Design review of the part built by this model. Coordinates are the model's own, in mm. Face numbers are marked on the shaded views. A direction names the side the tool comes from. Coordinates: 2 decimals unless noted, no trailing zeros. Order: outer loops, then holes, each group sorted by start corner. A loop starts at its lowest first (then second) coordinate and runs counter-clockwise, first axis right, second up. Notation, with made-up numbers: M 16.5,45 L 69.5,45 A16 cw 69.5,56 Z; hole C 45,-15.75 d8. An arc over 180 degrees is marked long. Use CSV: the item, a comma, the result in double quotes.
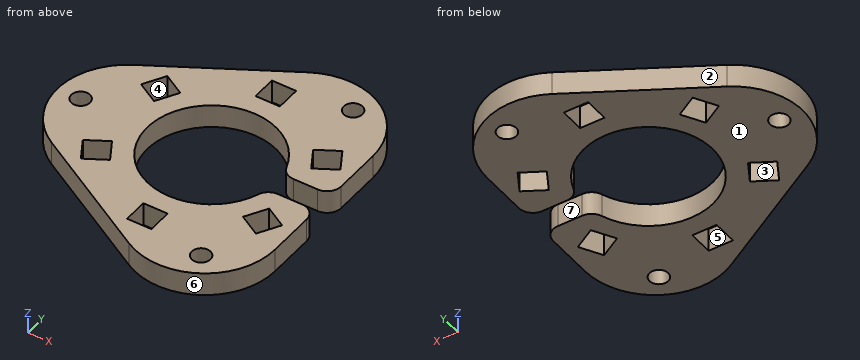
```python
from build123d import *

# Parameters (mm, degrees)
SKETCH1_R           = 2
SKETCH1_W           = 5.2
SKETCH1_H           = 5.2
BOSS_EXTRUDE1_DEPTH = 5
CONG_1_R            = 15
CONG_2_R            = 3


with BuildPart() as part:
    # Sketch1 → Boss-Extrude1 (new body)
    with BuildSketch(Plane.XY):
        with BuildLine():
            Line((24, 2.5), (13.520817283, 2.5))
            ThreePointArc((13.520817283, 2.5), (-13.75, 0), (13.520817283, -2.5))
            Line((13.520817283, -2.5), (24, -2.5))
            Line((24, -2.5), (24, -41.569219382))
            Line((24, -41.569219382), (-48, 0))
            Line((-48, 0), (24, 41.569219382))
            Line((24, 41.569219382), (24, 2.5))
        make_face()
        with Locations((14, 24.248711306)):
            Circle(SKETCH1_R, mode=Mode.SUBTRACT)
        with Locations((14, -24.248711306)):
            Circle(SKETCH1_R, mode=Mode.SUBTRACT)
        with Locations((-28, 0)):
            Circle(SKETCH1_R, mode=Mode.SUBTRACT)
        with Locations((0, 20.5)):
            Rectangle(SKETCH1_W, SKETCH1_H, mode=Mode.SUBTRACT)
        Polygon((21.305186827, 9.29833395), (16.801854728, 6.69833395), (14.201854728, 11.20166605), (18.705186827, 13.80166605), align=None, mode=Mode.SUBTRACT)
        Polygon((18.705186827, -13.80166605), (14.201854728, -11.20166605), (16.801854728, -6.69833395), (21.305186827, -9.29833395), align=None, mode=Mode.SUBTRACT)
        with Locations((0, -20.5)):
            Rectangle(SKETCH1_W, SKETCH1_H, mode=Mode.SUBTRACT)
        Polygon((-21.305186827, -9.29833395), (-16.801854728, -6.69833395), (-14.201854728, -11.20166605), (-18.705186827, -13.80166605), align=None, mode=Mode.SUBTRACT)
        Polygon((-18.705186827, 13.80166605), (-14.201854728, 11.20166605), (-16.801854728, 6.69833395), (-21.305186827, 9.29833395), align=None, mode=Mode.SUBTRACT)
    extrude(amount=BOSS_EXTRUDE1_DEPTH)

    # Congé1
    cong_1_edges = [part.edges().sort_by_distance(p)[0] for p in [
        (24, -41.569219382, 2.5),
        (-48, 0, 2.5),
        (24, 41.569219382, 2.5),
    ]]
    fillet(cong_1_edges, radius=CONG_1_R)

    # Congé2
    cong_2_edges = [part.edges().sort_by_distance(p)[0] for p in [
        (24, 2.5, 2.5),
        (13.520817283, 2.5, 2.5),
        (13.520817283, -2.5, 2.5),
        (24, -2.5, 2.5),
    ]]
    fillet(cong_2_edges, radius=CONG_2_R)


solid = part.part
```
(1) Add section B-B on x = 7.5. State the section outline as (y, z) points.
The answers:
outline,"M -30.51,0 L -11.52,0 L -11.52,5 L -30.51,5 Z; M 11.52,0 L 30.51,0 L 30.51,5 L 11.52,5 Z"
(2) Clearance check with flat-ended pins moving along their axes: P1, Ø2.5, axis at x = 1, z = 2, coming from the -Y side; P2, Ø1.5, axis at y = -20.5, z = 1.5, coming from the -X side; P3, Ø2.5, axis at x = 18.5, z = 3.5, coming from the -Y side; P4, Ø2.5, axis at x = 14, y = -24.25, coming from the +Z side. State where each tip first meets the part, or that it passes through.
The answers:
P1,"stops at y = -28.98"
P2,"stops at x = -13.79"
P3,"stops at y = -28.12"
P4,"passes through"
(3) Wall thickness on probe 1 along Y at (x, z) = (0, 1.95); probe 2 along Y at (x, z) = (-20.5, 2.6); probe 3 along Y at (x, z) = (17, 4.55): over which ranges is each line inside the solid? List them lowest first.
The answers:
probe 1,"y = -27.71 to -23.1, -17.9 to -13.75, 13.75 to 17.9, 23.1 to 27.71"
probe 2,"y = -15.88 to -10.69, -8.83 to 8.83, 10.69 to 15.88"
probe 3,"y = -28.28 to -12.82, -6.81 to -2.5, 2.5 to 6.81, 12.82 to 28.28"
(4) For the marked faces 5, 6 and 7, list the 3-axis set-ups (+Z, -Z, +X, -X, +Y, -Y) from which the entire face can be reached by the end or side of a thin tool; tool diameter is ignored.
The answers:
face 5,"+Z, -Z"
face 6,"+Z, -Z, -Y"
face 7,"+Z, -Z, +X"
(5) The part is to be moulded in two halves that separate along Y. For the marked faces 1, 2, 3 and 4, say which applies: pulls with the +Y half, pulls with the -Y half, needs draft (parallel to the pull), parting line crosses it, or undercut.
The answers:
face 1,"needs draft"
face 2,"pulls with the +Y half"
face 3,"undercut"
face 4,"undercut"
(6) Add section C-C on x = 0. State the section outline as (y, z) points.
The answers:
outline,"M -27.71,0 L -23.1,0 L -23.1,5 L -27.71,5 Z; M -17.9,0 L -13.75,0 L -13.75,5 L -17.9,5 Z; M 13.75,0 L 17.9,0 L 17.9,5 L 13.75,5 Z; M 23.1,0 L 27.71,0 L 27.71,5 L 23.1,5 Z"
(7) Add section D-D on z = 1.05. Give the number of separate pieces and of enclosed holes in the cut face, and give its area (3 significant figures).
The answers:
separate pieces,"1"
enclosed holes,"9"
area,"1,680 mm2"
(8) Add section A-A on y = 0. State the section outline as (x, z) points.
The answers:
outline,"M -33,0 L -30,0 L -30,5 L -33,5 Z; M -26,0 L -13.75,0 L -13.75,5 L -26,5 Z"
